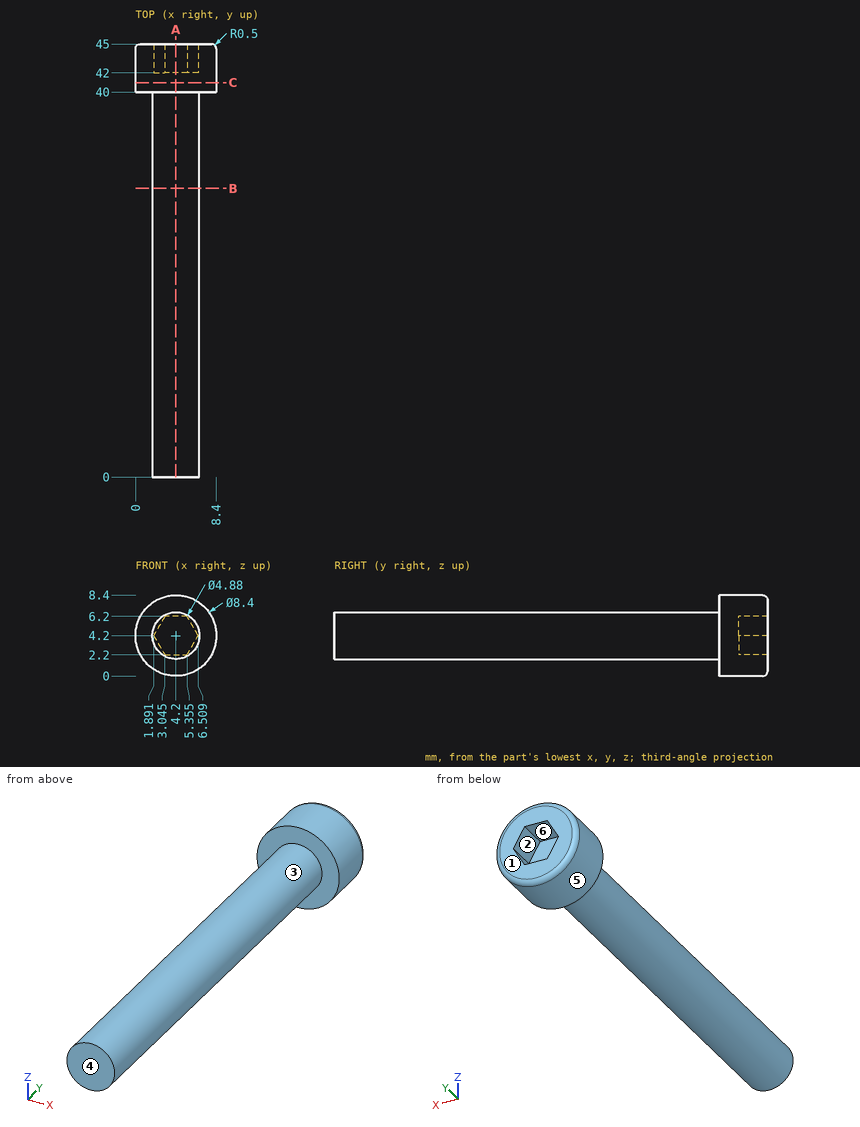
Geometry check sheet. Reference: drawing and pictorial views, mm from the part's lowest x, y, z. A direction names the side the tool comes from. Round coordinates to 2 decimals unless told otherwise and drop trailing zeros. Order: outer loops, then holes, each group sorted by start corner. A loop starts at its lowest first (then second) coordinate and runs counter-clockwise, first axis right, second up. Notation, with made-up numbers: M 31,88 L 84,88 A17 cw 84,105 Z; hole C -9.5,-2 d3. An arc over 180 degrees is marked long. Answer as CSV lines item,"result".
1) Tool access check on the marked faces 1, 2 and 3. Record the directions out of +Z, -Z, +X, -X, +Y, -Y that give a thin tool (end or side, any length) a straight path to the whole face; none if there is none.
Entries:
face 1,"+Z, -Z, +X, -X, +Y"
face 2,"+Y"
face 3,"-Y"
2) Mould release check, pull along Z, two halves, no side actions. Record for the marked faces 4, 5 and 6: +Z half, -Z half, draft (parallel to the pull), parting line (faces both ways), or undercut.
Entries:
face 4,"draft"
face 5,"parting line"
face 6,"undercut"
3) Sectioned sample at B-B on y = 30. Record the cut outline in (x, z).
Entries:
outline,"C 4.2,4.2 d4.88"
4) Gauge pin test, flat ends, axial feed: pin 1 Ø4 at (x, y) = (2, 36.5) entering from +Z; pin 2 Ø2 at (y, z) = (22, 2) entering from -X (1 decimal); pin 3 Ø5 at (y, z) = (13, 2.5) entering from +X. Record the tip position at first contact, or that the pin passes through.
Entries:
pin 1,"z = 6.63"
pin 2,"x = 2.1"
pin 3,"x = 6.64"
5) Thickness scan on probe 1 along Y at (x, z) = (3.5, 1.25); probe 2 along Y at (x, z) = (3.75, 5); probe 3 along Z at (x, y) = (2, 24.5) (1 decimal). Record the ranges inside material, lowest first. Write a range as [from, to].
Entries:
probe 1,"[40, 45]"
probe 2,"[0, 42]"
probe 3,"[3.1, 5.3]"
6) Sectioned sample at C-C on y = 41. Record the cut outline in (x, z).
Entries:
outline,"C 4.2,4.2 d8.4"
7) Sectioned sample at A-A on x = 4.2. Record the cut outline in (y, z).
Entries:
outline,"M 0,1.76 L 40,1.76 L 40,0 L 44.5,0 A0.5 ccw 45,0.5 L 45,2.2 L 42,2.2 L 42,6.2 L 45,6.2 L 45,7.9 A0.5 ccw 44.5,8.4 L 40,8.4 L 40,6.64 L 0,6.64 Z"
